Autodesk Inventor part; units mm, degrees
ref_plane "body_to_body_c_XY" through (0, 12.8016, 0) normal (0, -1, 0) x (1, 0, 0)
ref_plane "body_to_body_c_YZ" through (0, 12.8016, 0) normal (1, 0, 0) x (0, 0, 1)
ref_plane "body_to_body_c_ZX" through (0, 12.8016, 0) normal (0, 0, 1) x (0, -1, 0)
sketch "Sketch_1" plane through (0, 0, 0) normal (1, 0, 0) x (0, 1, 0)
  line L0 (12.8016, 6.5024) -> (0, 6.5024)
  line L1 (0, 6.5024) -> (0, -6.5024)
  line L2 (0, -6.5024) -> (12.8016, -6.5024)
  line L3 (12.8016, -6.5024) -> (12.8016, 6.5024)
extrude "Extrusion1" add sketch "Sketch_1" along normal mid plane 12.7
sketch "Sketch_5" plane through (6.35, 0, 0) normal (1, 0, 0) x (0, 0, -1)
  line L0 (-6.5024, 9.7536) -> (-5.4864, 9.7536)
  arc A0 (-4.9784, 9.2456) -> (-5.4864, 9.7536) centre (-5.4864, 9.2456) ccw
  line L1 (-4.9784, 9.2456) -> (-4.9784, 0)
  line L2 (-4.9784, 0) -> (4.9784, 0)
  line L3 (4.9784, 0) -> (4.9784, 9.2456)
  arc A1 (5.4864, 9.7536) -> (4.9784, 9.2456) centre (5.4864, 9.2456) ccw
  line L4 (5.4864, 9.7536) -> (6.5024, 9.7536)
  line L5 (6.5024, 9.7536) -> (6.5024, 13.0556)
  line L6 (6.5024, 13.0556) -> (-6.5024, 13.0556)
  line L7 (-6.5024, 13.0556) -> (-6.5024, 9.7536)
extrude "Extrusion2" cut sketch "Sketch_5" against normal blind 0.254
sketch "Sketch_6" plane through (-6.35, 0, 0) normal (1, 0, 0) x (0, 0, -1)
  line L0 (-6.5024, 9.7536) -> (-5.4864, 9.7536)
  arc A0 (-4.9784, 9.2456) -> (-5.4864, 9.7536) centre (-5.4864, 9.2456) ccw
  line L1 (-4.9784, 9.2456) -> (-4.9784, 0)
  line L2 (-4.9784, 0) -> (4.9784, 0)
  line L3 (4.9784, 0) -> (4.9784, 9.2456)
  arc A1 (5.4864, 9.7536) -> (4.9784, 9.2456) centre (5.4864, 9.2456) ccw
  line L4 (5.4864, 9.7536) -> (6.5024, 9.7536)
  line L5 (6.5024, 9.7536) -> (6.5024, 13.0556)
  line L6 (6.5024, 13.0556) -> (-6.5024, 13.0556)
  line L7 (-6.5024, 13.0556) -> (-6.5024, 9.7536)
extrude "Extrusion3" cut sketch "Sketch_6" along normal blind 0.254
sketch "Sketch_7" plane through (0, 0, -6.5024) normal (0, 0, 1) x (1, 0, 0)
  line L0 (-6.35, 9.7536) -> (6.35, 9.7536)
  line L1 (6.35, 9.7536) -> (6.35, 13.0556)
  line L2 (6.35, 13.0556) -> (-6.35, 13.0556)
  line L3 (-6.35, 13.0556) -> (-6.35, 9.7536)
extrude "Extrusion4" cut sketch "Sketch_7" along normal blind 0.254
sketch "Sketch_8" plane through (0, 0, 6.5024) normal (0, 0, 1) x (1, 0, 0)
  line L0 (-6.35, 9.7536) -> (6.35, 9.7536)
  line L1 (6.35, 9.7536) -> (6.35, 13.0556)
  line L2 (6.35, 13.0556) -> (-6.35, 13.0556)
  line L3 (-6.35, 13.0556) -> (-6.35, 9.7536)
extrude "Extrusion5" cut sketch "Sketch_8" against normal blind 0.254
sketch "Sketch_9" plane through (0, 0, 0) normal (0, 1, 0) x (-1, 0, 0)
  line L0 (8.128, 8.2804) -> (-8.128, 8.2804)
  line L1 (-8.128, 8.2804) -> (-8.128, -8.2804)
  line L2 (-8.128, -8.2804) -> (8.128, -8.2804)
  line L3 (8.128, -8.2804) -> (8.128, 8.2804)
  line L4 (6.35, -1.5875) -> (6.35, 1.5875)
  line L5 (6.35, 1.5875) -> (5.08, 1.8415)
  line L6 (5.08, 1.8415) -> (5.08, 2.8575)
  line L7 (5.08, 2.8575) -> (6.35, 3.1115)
  line L8 (6.35, 3.1115) -> (6.35, 6.5024)
  line L9 (6.35, 6.5024) -> (-6.35, 6.5024)
  line L10 (-6.35, 6.5024) -> (-6.35, 3.1115)
  line L11 (-6.35, 3.1115) -> (-5.08, 2.8575)
  line L12 (-5.08, 2.8575) -> (-5.08, 1.8415)
  line L13 (-5.08, 1.8415) -> (-6.35, 1.5875)
  line L14 (-6.35, 1.5875) -> (-6.35, -1.5875)
  line L15 (-6.35, -1.5875) -> (-5.08, -1.8415)
  line L16 (-5.08, -1.8415) -> (-5.08, -2.8575)
  line L17 (-5.08, -2.8575) -> (-6.35, -3.1115)
  line L18 (-6.35, -3.1115) -> (-6.35, -6.5024)
  line L19 (-6.35, -6.5024) -> (6.35, -6.5024)
  line L20 (6.35, -6.5024) -> (6.35, -3.1115)
  line L21 (6.35, -3.1115) -> (5.08, -2.8575)
  line L22 (5.08, -2.8575) -> (5.08, -1.8415)
  line L23 (5.08, -1.8415) -> (6.35, -1.5875)
extrude "Extrusion6" cut sketch "Sketch_9" along normal blind 2.54
sketch "Sketch_10" plane through (0, 0, 0) normal (0, 0, 1) x (1, 0, 0)
  line L0 (-0.381, 0) -> (-0.381, -1.1684)
  arc A0 (-0.381, -1.1684) -> (0.381, -1.1684) centre (0, -1.1684) ccw
  line L1 (0.381, -1.1684) -> (0.381, 0)
  line L2 (0.381, 0) -> (-0.381, 0)
extrude "Extrusion7" add sketch "Sketch_10" along normal mid plane 11.43
sketch "Sketch_11" plane through (0, 0, 0) normal (1, 0, 0) x (0, 1, 0)
  arc A0 (-0.381, 2.7305) -> (-0.381, 1.9685) centre (-0.381, 2.3495) ccw
  line L0 (-0.381, 1.9685) -> (0, 1.9685)
  line L1 (0, 1.9685) -> (0, -1.9685)
  line L2 (0, -1.9685) -> (-0.381, -1.9685)
  arc A1 (-0.381, -1.9685) -> (-0.381, -2.7305) centre (-0.381, -2.3495) ccw
  line L3 (-0.381, -2.7305) -> (0.508, -2.7305)
  line L4 (0.508, -2.7305) -> (0.508, 2.7305)
  line L5 (0.508, 2.7305) -> (-0.381, 2.7305)
extrude "Extrusion8" add sketch "Sketch_11" along normal mid plane 9.144
ref_plane "body_to_body_c_XY" through (0, 12.8016, 0) normal (0, -1, 0) x (1, 0, 0)
ref_plane "body_to_body_c_YZ" through (0, 12.8016, 0) normal (1, 0, 0) x (0, 0, 1)
ref_plane "body_to_body_c_ZX" through (0, 12.8016, 0) normal (0, 0, 1) x (0, -1, 0)
ref_plane "body_to_dummy_XY" through (0, 0, 0) normal (0, -1, 0) x (1, 0, 0)
ref_plane "body_to_dummy_YZ" through (0, 0, 0) normal (1, 0, 0) x (0, 0, 1)
ref_plane "body_to_dummy_ZX" through (0, 0, 0) normal (0, 0, 1) x (0, -1, 0)
ref_plane "body_to_terminal_XY" through (0, 0, 0) normal (0, -1, 0) x (1, 0, 0)
ref_plane "body_to_terminal_YZ" through (0, 0, 0) normal (1, 0, 0) x (0, 0, 1)
ref_plane "body_to_terminal_ZX" through (0, 0, 0) normal (0, 0, 1) x (0, -1, 0)
properties part number "M211LW01-body"
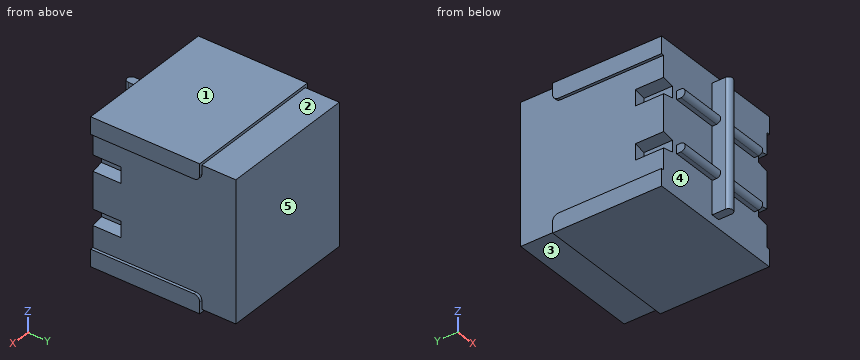
Work out the finished part from the listing and answer in its coordinate system (mm). Face numbers are marked on the shaded views. A direction names the side the tool comes from. Round coordinates to 2 decimals unless told otherwise and drop trailing zeros. Loops run counter-clockwise (first coordinate to the right, second up) from the corner with the lowest first, then second, coordinate; pieces in that order, holes last. Notation, with made-up numbers: (61.25, -23.75) -> (65.25, -23.75) arc R13 cw to (65.25, -0.75) -> close; hole circle Ø4 at (-18.75, 19). An arc over 180 degrees is marked (long way). Use one line per item in the form item = value.
(1) A tool of negligible diameter and unlimited length cuts with its end or side. For the marked faces 1 and 2, from which of +Z, -Z, +X, -X, +Y, -Y can it reach the whole face along a straight path? Write none if from no direction.
Answer list:
face_1 = +Z, +X, -X, +Y, -Y
face_2 = +Z, +X, -X, +Y
(2) Straight lines are drawn through the part: line 1 (X direction, y = 3, z = -1); line 2 (Y direction, x = -0.75, z = 4.5); line 3 (Z direction, x = -5.5, y = 12.25). For each, find the intervals that lie inside material, in ascending order.
Answer list:
line_1 = -6.1 to 6.1
line_2 = 0 to 12.8
line_3 = -6.25 to 6.25
(3) Find section B-B on y = 4. Give the vertices of the cut face in (x, z).
Answer list:
outline = (-6.35, -6.5) -> (6.35, -6.5) -> (6.35, -4.98) -> (6.1, -4.98) -> (6.1, 4.98) -> (6.35, 4.98) -> (6.35, 6.5) -> (-6.35, 6.5) -> (-6.35, 4.98) -> (-6.1, 4.98) -> (-6.1, -4.98) -> (-6.35, -4.98) -> close
(4) For a pull along Z with two mould halves and no side action, classify the marked faces 3, 4 and 5 as released by +Z, released by -Z, zero draft, split by the parting line, or undercut.
Answer list:
face_3 = released by -Z
face_4 = undercut
face_5 = zero draft
(5) Flat-ended cylindrical pins translate along their axes: P1, Ø0.6, axis at y = -0.5, z = -2, coming from the -X side; P2, Ø6, axis at y = 1.5, z = 0.5, coming from the +X side; P3, Ø5, axis at x = -4, z = 3, coming from the -Y side. Find the tip coordinate at first contact, or state that the pin passes through.
Answer list:
P1 = -4.57
P2 = 6.1
P3 = -0.76
(6) Find section C-C on x = 1. Give the vertices of the cut face in (y, z), then the cut area to 3 significant figures.
Answer list:
outline = (-0.38, -2.73) -> (0, -2.73) -> (0, -6.5) -> (9.75, -6.5) -> (9.75, -6.25) -> (12.8, -6.25) -> (12.8, 6.25) -> (9.75, 6.25) -> (9.75, 6.5) -> (0, 6.5) -> (0, 2.73) -> (-0.38, 2.73) arc R0.38 ccw to (-0.38, 1.97) -> (0, 1.97) -> (0, -1.97) -> (-0.38, -1.97) arc R0.38 ccw to start
area = 166 mm2
(7) Find section D-D on y = 2. Give the vertices of the cut face in (x, z).
Answer list:
outline = (-6.35, -6.5) -> (6.35, -6.5) -> (6.35, -4.98) -> (6.1, -4.98) -> (6.1, -3.06) -> (5.08, -2.86) -> (5.08, -1.84) -> (6.1, -1.64) -> (6.1, 1.64) -> (5.08, 1.84) -> (5.08, 2.86) -> (6.1, 3.06) -> (6.1, 4.98) -> (6.35, 4.98) -> (6.35, 6.5) -> (-6.35, 6.5) -> (-6.35, 4.98) -> (-6.1, 4.98) -> (-6.1, 3.06) -> (-5.08, 2.86) -> (-5.08, 1.84) -> (-6.1, 1.64) -> (-6.1, -1.64) -> (-5.08, -1.84) -> (-5.08, -2.86) -> (-6.1, -3.06) -> (-6.1, -4.98) -> (-6.35, -4.98) -> close
(8) Find section A-A on z = 0.75. Give the vertices of the cut face in (x, y), then the cut area to 3 significant figures.
Answer list:
outline = (-6.1, 0) -> (-0.38, 0) -> (-0.38, -1.17) arc R0.38 ccw to (0.38, -1.17) -> (0.38, 0) -> (6.1, 0) -> (6.1, 12.8) -> (-6.1, 12.8) -> close
area = 157 mm2
